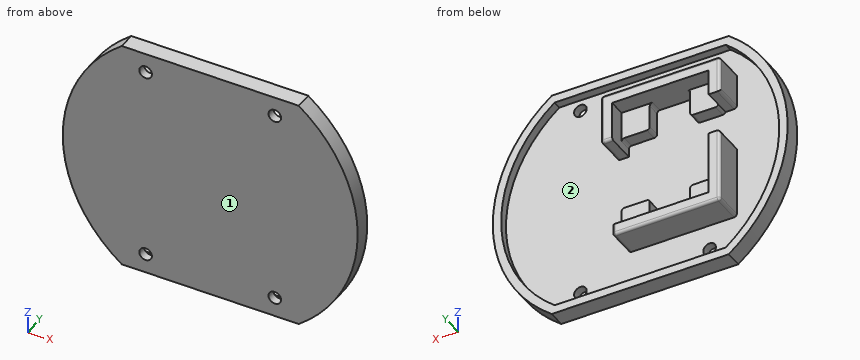
from build123d import *

# Parameters (mm, degrees)
A_BASE_T42_OUTLINE_R       = 2.2479
A_BASE_T42_OUTLINE_R_2     = 1
A_BASE_T42_DEPTH           = 3
OUTER_BRIM_DEPTH           = 3
SKETCH5_W                  = 3
SKETCH5_H                  = 15
SKETCH5_W_2                = 15
SKETCH5_H_2                = 3
BASE_SUPPORTS_DEPTH        = 3
BASE_SUPPORTS_CHAMFER_SIZE = 3
COVER_START                = -3
SKETCH6_R                  = 1
COVER_DEPTH                = 3
SKETCH9_W                  = 15
SKETCH9_H                  = 6
SKETCH9_W_2                = 6
SKETCH9_H_2                = 15
CUT_EXTRUDE1_DEPTH         = 10
SKETCH10_W                 = 10
SKETCH10_H                 = 10
BOSS_EXTRUDE1_DEPTH        = 4.6
BOSS_EXTRUDE2_DEPTH        = 10.6
FILLET1_R                  = 1


with BuildPart() as part:
    # a_base_t42: read off the stored shape, not the designer's step
    # a_base_t42 outline → a_base_t42 (new body)
    with BuildSketch(Plane(origin=(0, 0, 0), x_dir=(1, 0, 0), z_dir=(0, 1, 0))):
        with BuildLine():
            ThreePointArc((31.5, -42), (52.5, 0), (31.5, 42))
            Line((31.5, 42), (-31.5, 42))
            ThreePointArc((-31.5, 42), (-52.5, 0), (-31.5, -42))
            Line((-31.5, -42), (31.5, -42))
        make_face()
        with Locations((-23, -35)):
            Circle(A_BASE_T42_OUTLINE_R, mode=Mode.SUBTRACT)
        with Locations((23, -35)):
            Circle(A_BASE_T42_OUTLINE_R, mode=Mode.SUBTRACT)
        with Locations((-40.25, 0)):
            Circle(A_BASE_T42_OUTLINE_R_2, mode=Mode.SUBTRACT)
        with Locations((-23, 35)):
            Circle(A_BASE_T42_OUTLINE_R, mode=Mode.SUBTRACT)
        with Locations((40.25, 0)):
            Circle(A_BASE_T42_OUTLINE_R_2, mode=Mode.SUBTRACT)
        with Locations((23, 35)):
            Circle(A_BASE_T42_OUTLINE_R, mode=Mode.SUBTRACT)
    extrude(amount=A_BASE_T42_DEPTH)

    # Sketch1 → Outer Brim (add)
    with BuildSketch(Plane(origin=(0, 3, 0), x_dir=(1, 0, 0), z_dir=(0, 1, 0))):
        with BuildLine():
            Line((-31.5, -42), (31.5, -42))
            ThreePointArc((31.5, -42), (52.5, 0), (31.5, 42))
            Line((31.5, 42), (-31.5, 42))
            ThreePointArc((-31.5, 42), (-52.5, 0), (-31.5, -42))
        make_face()
        with BuildLine():
            Line((30.483602149, 39), (-30.483602149, 39))
            ThreePointArc((-30.483602149, 39), (-49.5, 0), (-30.483602149, -39))
            Line((-30.483602149, -39), (30.483602149, -39))
            ThreePointArc((30.483602149, -39), (49.5, 0), (30.483602149, 39))
        make_face(mode=Mode.SUBTRACT)
    extrude(amount=OUTER_BRIM_DEPTH)

    # Sketch5 → Base Supports (add)
    with BuildSketch(Plane(origin=(0, 3, 0), x_dir=(1, 0, 0), z_dir=(0, 1, 0))):
        with Locations((-34.325, -12.5)):
            Rectangle(SKETCH5_W, SKETCH5_H)
        with Locations((-34.325, 12.5)):
            Rectangle(SKETCH5_W, SKETCH5_H)
        with Locations((-25.325, -27)):
            Rectangle(SKETCH5_W_2, SKETCH5_H_2)
        with Locations((-25.325, 27)):
            Rectangle(SKETCH5_W_2, SKETCH5_H_2)
    extrude(amount=BASE_SUPPORTS_DEPTH)

    # Base Supports Chamfer
    base_supports_chamfer_edges = [part.edges().sort_by_distance(p)[0] for p in [
        (-25.325, 3, 28.5),
        (-25.325, 3, -28.5),
        (-35.825, 3, 12.5),
        (-35.825, 3, -12.5),
    ]]
    chamfer(base_supports_chamfer_edges, length=BASE_SUPPORTS_CHAMFER_SIZE - 0.0001)  # a hair under: the kernel refuses the full size

    # Sketch6 → Cover (add)
    with BuildSketch(Plane(origin=(0, 3, 0), x_dir=(1, 0, 0), z_dir=(0, 1, 0)).offset(COVER_START)):
        with Locations((-40.25, 0)):
            Circle(SKETCH6_R)
        with Locations((40.25, 0)):
            Circle(SKETCH6_R)
    extrude(amount=COVER_DEPTH)

    # Sketch9 → Cut-Extrude1 (cut)
    with BuildSketch(Plane(origin=(0, 3, 0), x_dir=(1, 0, 0), z_dir=(0, 1, 0))):
        with Locations((-25.325, 28.5)):
            Rectangle(SKETCH9_W, SKETCH9_H)
        with Locations((-35.825, 12.5)):
            Rectangle(SKETCH9_W_2, SKETCH9_H_2)
        with Locations((-35.825, -12.5)):
            Rectangle(SKETCH9_W_2, SKETCH9_H_2)
        with Locations((-25.325, -28.5)):
            Rectangle(SKETCH9_W, SKETCH9_H)
    extrude(amount=CUT_EXTRUDE1_DEPTH, mode=Mode.SUBTRACT)

    # Sketch10 → Boss-Extrude1 (add)
    with BuildSketch(Plane(origin=(0, 3, 0), x_dir=(1, 0, 0), z_dir=(0, 1, 0))):
        with Locations((-23.7, 16.95)):
            Rectangle(SKETCH10_W, SKETCH10_H)
        with Locations((0.7, 16.95)):
            Rectangle(SKETCH10_W, SKETCH10_H)
        with Locations((0.7, -19.95)):
            Rectangle(SKETCH10_W, SKETCH10_H)
        with Locations((-23.7, -19.95)):
            Rectangle(SKETCH10_W, SKETCH10_H)
    extrude(amount=BOSS_EXTRUDE1_DEPTH)

    # Sketch11 → Boss-Extrude2 (add)
    with BuildSketch(Plane(origin=(0, 3, 0), x_dir=(1, 0, 0), z_dir=(0, 1, 0))):
        Polygon((-28.7, 21.95), (-28.7, -0.7), (-32.7, -0.7), (-32.7, 25.95), (5.7, 25.95), (5.7, 21.95), align=None)
        Polygon((-28.7, -24.95), (-28.7, -15.7), (-32.7, -15.7), (-32.7, -28.95), (9.7, -28.95), (9.7, -10.95), (5.7, -10.95), (5.7, -24.95), align=None)
    extrude(amount=BOSS_EXTRUDE2_DEPTH)

    # Fillet1
    # the kernel refuses this fillet: 1 mm, written as the material it adds along each edge
    with BuildSketch(Plane(origin=(-18.7, 0.5, 24.95), x_dir=(1, 0, 0), z_dir=(0, 1, 0)), Plane(origin=(-4.3, 0.5, 24.95), x_dir=(0, 0, -1), z_dir=(0, 1, 0)), Plane(origin=(5.7, 0.5, 14.95), x_dir=(0, 0, -1), z_dir=(0, 1, 0)), Plane(origin=(-4.3, 0.5, -21.95), x_dir=(-1, 0, 0), z_dir=(0, 1, 0)), Plane(origin=(-18.7, 0.5, -21.95), x_dir=(0, 0, 1), z_dir=(0, 1, 0)), Plane(origin=(-28.7, 0.5, -11.95), x_dir=(0, 0, 1), z_dir=(0, 1, 0))) as fillet1_piece_1:
        with BuildLine():
            CenterArc((FILLET1_R, FILLET1_R), FILLET1_R, 180, 90)
            Line((0, FILLET1_R), (0, 0))
            Line((0, 0), (FILLET1_R, 0))
        make_face()
    extrude(amount=7.1)
    # the kernel refuses this fillet: 1 mm, written as the material it takes off along each edge
    with BuildSketch(Plane(origin=(-31.7, 12.6, 27.95), x_dir=(0, 1, 0), z_dir=(-1, 0, 0))) as fillet1_2_piece_1_section:
        Polygon((0, 0), (FILLET1_R * 1.02, 0), (FILLET1_R * 1.02, -FILLET1_R * 1.02), (0, -FILLET1_R * 1.02), align=None)
    fillet1_2_piece_1 = extrude(amount=FILLET1_R * 1.02, mode=Mode.PRIVATE)
    fillet1_2_piece_1 = fillet1_2_piece_1 - Plane(origin=(-31.7, 12.6, 27.95), x_dir=(0, -0.7071067811865475, -0.7071067811865475), z_dir=(-1, 0, 0)) * Sphere(FILLET1_R, mode=Mode.PRIVATE)
    add(fillet1_2_piece_1, mode=Mode.SUBTRACT)
    with BuildSketch(Plane(origin=(8.7, 12.6, 27.95), x_dir=(1, 0, 0), z_dir=(0, 1, 0))) as fillet1_2_piece_2_section:
        Polygon((0, 0), (FILLET1_R * 1.02, 0), (FILLET1_R * 1.02, -FILLET1_R * 1.02), (0, -FILLET1_R * 1.02), align=None)
    fillet1_2_piece_2 = extrude(amount=FILLET1_R * 1.02, mode=Mode.PRIVATE)
    fillet1_2_piece_2 = fillet1_2_piece_2 - Plane(origin=(8.7, 12.6, 27.95), x_dir=(-0.7071067811865475, 0, -0.7071067811865475), z_dir=(0, 1, 0)) * Sphere(FILLET1_R, mode=Mode.PRIVATE)
    add(fillet1_2_piece_2, mode=Mode.SUBTRACT)
    with BuildSketch(Plane(origin=(8.7, 12.6, 11.95), x_dir=(0, 1, 0), z_dir=(0, 0, -1))) as fillet1_2_piece_3_section:
        Polygon((0, 0), (FILLET1_R * 1.02, 0), (FILLET1_R * 1.02, FILLET1_R * 1.02), (0, FILLET1_R * 1.02), align=None)
    fillet1_2_piece_3 = extrude(amount=FILLET1_R * 1.02, mode=Mode.PRIVATE)
    fillet1_2_piece_3 = fillet1_2_piece_3 - Plane(origin=(8.7, 12.6, 11.95), x_dir=(-0.7071067811865475, -0.7071067811865475, 0), z_dir=(0, 0, -1)) * Sphere(FILLET1_R, mode=Mode.PRIVATE)
    add(fillet1_2_piece_3, mode=Mode.SUBTRACT)
    with BuildSketch(Plane(origin=(4.7, 12.6, -24.95), x_dir=(1, 0, 0), z_dir=(0, 0, -1))) as fillet1_2_piece_4_section:
        Polygon((0, 0), (FILLET1_R * 1.02, 0), (FILLET1_R * 1.02, -FILLET1_R * 1.02), (0, -FILLET1_R * 1.02), align=None)
    fillet1_2_piece_4 = extrude(amount=FILLET1_R * 1.02, mode=Mode.PRIVATE)
    fillet1_2_piece_4 = fillet1_2_piece_4 - Plane(origin=(4.7, 12.6, -24.95), x_dir=(-0.7071067811865475, -0.7071067811865475, 0), z_dir=(0, 0, -1)) * Sphere(FILLET1_R, mode=Mode.PRIVATE)
    add(fillet1_2_piece_4, mode=Mode.SUBTRACT)
    with BuildSketch(Plane(origin=(-31.7, 12.6, -24.95), x_dir=(0, 1, 0), z_dir=(0, 0, -1))) as fillet1_2_piece_5_section:
        Polygon((0, 0), (FILLET1_R * 1.02, 0), (FILLET1_R * 1.02, -FILLET1_R * 1.02), (0, -FILLET1_R * 1.02), align=None)
    fillet1_2_piece_5 = extrude(amount=FILLET1_R * 1.02, mode=Mode.PRIVATE)
    fillet1_2_piece_5 = fillet1_2_piece_5 - Plane(origin=(-31.7, 12.6, -24.95), x_dir=(0.7071067811865475, -0.7071067811865475, 0), z_dir=(0, 0, -1)) * Sphere(FILLET1_R, mode=Mode.PRIVATE)
    add(fillet1_2_piece_5, mode=Mode.SUBTRACT)
    with BuildSketch(Plane(origin=(-32.7, 13.6, 13.2), x_dir=(1, 0, 0), z_dir=(0, 0, 1))) as fillet1_2_piece_6:
        with BuildLine():
            CenterArc((FILLET1_R, -FILLET1_R), FILLET1_R, 90, 90)
            Line((0, -FILLET1_R), (0, 0))
            Line((0, 0), (FILLET1_R, 0))
        make_face()
    extrude(amount=14.75, mode=Mode.SUBTRACT)
    with BuildSketch(Plane(origin=(-31.7, 13.6, 28.95), x_dir=(0, 0, -1), z_dir=(1, 0, 0))) as fillet1_2_piece_7:
        with BuildLine():
            CenterArc((FILLET1_R, -FILLET1_R), FILLET1_R, 90, 90)
            Line((0, -FILLET1_R), (0, 0))
            Line((0, 0), (FILLET1_R, 0))
        make_face()
    extrude(amount=40.4, mode=Mode.SUBTRACT)
    with BuildSketch(Plane(origin=(9.7, 13.6, 27.95), x_dir=(-1, 0, 0), z_dir=(0, 0, -1))) as fillet1_2_piece_8:
        with BuildLine():
            CenterArc((FILLET1_R, -FILLET1_R), FILLET1_R, 90, 90)
            Line((0, -FILLET1_R), (0, 0))
            Line((0, 0), (FILLET1_R, 0))
        make_face()
    extrude(amount=16, mode=Mode.SUBTRACT)
    with BuildSketch(Plane(origin=(5.7, 13.6, -24.95), x_dir=(-1, 0, 0), z_dir=(0, 0, 1))) as fillet1_2_piece_9:
        with BuildLine():
            CenterArc((FILLET1_R, FILLET1_R), FILLET1_R, 180, 90)
            Line((0, FILLET1_R), (0, 0))
            Line((0, 0), (FILLET1_R, 0))
        make_face()
    extrude(amount=5.5, mode=Mode.SUBTRACT)
    with BuildSketch(Plane(origin=(-31.7, 13.6, -25.95), x_dir=(0, 0, 1), z_dir=(1, 0, 0))) as fillet1_2_piece_10:
        with BuildLine():
            CenterArc((FILLET1_R, FILLET1_R), FILLET1_R, 180, 90)
            Line((0, FILLET1_R), (0, 0))
            Line((0, 0), (FILLET1_R, 0))
        make_face()
    extrude(amount=36.4, mode=Mode.SUBTRACT)
    with BuildSketch(Plane(origin=(-32.7, 13.6, 3.2), x_dir=(1, 0, 0), z_dir=(0, 0, -1))) as fillet1_2_piece_11:
        with BuildLine():
            CenterArc((FILLET1_R, FILLET1_R), FILLET1_R, 180, 90)
            Line((0, FILLET1_R), (0, 0))
            Line((0, 0), (FILLET1_R, 0))
        make_face()
    extrude(amount=28.15, mode=Mode.SUBTRACT)
    with BuildSketch(Plane(origin=(-32.7, 3, 0.7), x_dir=(1, 0, 0), z_dir=(0, 1, 0)), Plane(origin=(-32.7, 3, 15.7), x_dir=(0, 0, 1), z_dir=(0, 1, 0))) as fillet1_2_piece_12:
        with BuildLine():
            CenterArc((FILLET1_R, FILLET1_R), FILLET1_R, 180, 90)
            Line((0, FILLET1_R), (0, 0))
            Line((0, 0), (FILLET1_R, 0))
        make_face()
    extrude(amount=13.1, mode=Mode.SUBTRACT)
    with BuildSketch(Plane(origin=(-32.7, 3, -25.95), x_dir=(0, 0, 1), z_dir=(0, 1, 0)), Plane(origin=(5.7, 3, -25.95), x_dir=(-1, 0, 0), z_dir=(0, 1, 0)), Plane(origin=(9.7, 3, 10.95), x_dir=(-1, 0, 0), z_dir=(0, 1, 0)), Plane(origin=(9.7, 3, 28.95), x_dir=(0, 0, -1), z_dir=(0, 1, 0)), Plane(origin=(-32.7, 3, 28.95), x_dir=(1, 0, 0), z_dir=(0, 1, 0))) as fillet1_2_piece_13:
        with BuildLine():
            CenterArc((FILLET1_R, FILLET1_R), FILLET1_R, 180, 90)
            Line((0, FILLET1_R), (0, 0))
            Line((0, 0), (FILLET1_R, 0))
        make_face()
    extrude(amount=9.6, mode=Mode.SUBTRACT)
    with BuildSketch(Plane(origin=(-28.7, 3, 14.95), x_dir=(0, 0, 1), z_dir=(0, 1, 0))) as fillet1_2_piece_14:
        with BuildLine():
            CenterArc((1, 0.968245837), FILLET1_R, 180, 75.522487814)
            Line((0, 0.968245837), (0, 0))
            Line((0, 0), (0.75, 0))
        make_face()
    extrude(amount=7.020614591, mode=Mode.SUBTRACT)
    with BuildSketch(Plane(origin=(-18.7, 3, 14.95), x_dir=(-1, 0, 0), z_dir=(0, 1, 0)), Plane(origin=(-4.3, 3, 14.95), x_dir=(0, 0, 1), z_dir=(0, 1, 0)), Plane(origin=(5.7, 3, -11.95), x_dir=(0, 0, -1), z_dir=(0, 1, 0)), Plane(origin=(-4.3, 3, -11.95), x_dir=(1, 0, 0), z_dir=(0, 1, 0))) as fillet1_2_piece_15:
        with BuildLine():
            CenterArc((FILLET1_R, FILLET1_R), FILLET1_R, 180, 90)
            Line((0, FILLET1_R), (0, 0))
            Line((0, 0), (FILLET1_R, 0))
        make_face()
    extrude(amount=7.1, mode=Mode.SUBTRACT)
    with BuildSketch(Plane(origin=(-18.7, 3, -11.95), x_dir=(-1, 0, 0), z_dir=(0, 1, 0))) as fillet1_2_piece_16:
        with BuildLine():
            CenterArc((FILLET1_R, -FILLET1_R), FILLET1_R, 90, 90)
            Line((0, -FILLET1_R), (0, 0))
            Line((0, 0), (FILLET1_R, 0))
        make_face()
    extrude(amount=7.1, mode=Mode.SUBTRACT)
    with BuildSketch(Plane(origin=(8.7, 13.6, 10.95), x_dir=(0, 0, 1), z_dir=(-1, 0, 0))) as fillet1_2_piece_17:
        with BuildLine():
            CenterArc((FILLET1_R, -FILLET1_R), FILLET1_R, 90, 90)
            Line((0, -FILLET1_R), (0, 0))
            Line((0, 0), (FILLET1_R, 0))
        make_face()
    extrude(amount=5.5, mode=Mode.SUBTRACT)


solid = part.part
Geometry check sheet. Reference: the model listing, model coordinates, mm. Face numbers are marked on the shaded views. Round coordinates to 2 decimals unless told otherwise and drop trailing zeros. Write each loop counter-clockwise with the first axis right and the second up, starting at its lowest first coordinate (ties: lowest second). Pieces come first, ordered by that corner, then holes. Notation, with made-up numbers: (77.25, 10) - (123.25, 10) arc R27 ccw to (123.25, 40) - close; hole circle Ø8 at (49.25, -3). An arc over 180 degrees is marked (long way). One line per item, written item: value.
1. Cross-section at B-B on x = 23. Record the boundary of the cut face in (y, z), and give its area (3 significant figures).
The answers:
outline: (0, -42) - (6, -42) - (6, -39) - (3, -39) - (3, -37.25) - (0, -37.25) - close; (0, -32.75) - (3, -32.75) - (3, 32.75) - (0, 32.75) - close; (0, 37.25) - (3, 37.25) - (3, 39) - (6, 39) - (6, 42) - (0, 42) - close
area: 243 mm^2
2. Scan lines: L1, parallel to Z at x = 23, y = 2; L2, parallel to Z at x = 4, y = 5.5; L3, parallel to Z at x = -8.5, y = 11. Record each from-to range of solid material in increasing order.
The answers:
L1: z = -42 to -37.25, -32.75 to 32.75, 37.25 to 42
L2: z = -42 to -39, -25.95 to -11.95, 14.95 to 28.95, 39 to 42
L3: z = -25.95 to -21.95, 24.95 to 28.95
3. Depth check by flat-ended pin: pin 1 Ø5 at (y, z) = (7.5, -14) entering from -X; pin 2 Ø4 at (y, z) = (6, -12.5) entering from +X; pin 3 Ø1 at (y, z) = (2, -26.5) entering from +X. Enter the tip coordinate at first touch or a pass-through.
The answers:
pin 1: stops at x = -51.11
pin 2: stops at x = 51.44
pin 3: stops at x = 45.61
4. Cross-section at C-C on y = 4.75. Give the number of separate pieces and of enclosed holes in the cut face, and give its area (3 significant figures).
The answers:
separate pieces: 3
enclosed holes: 1
area: 1,840 mm^2
5. Cross-section at D-D on z = 35. Record the boundary of the cut face in (x, y).
The answers:
outline: (-39.13, 0) - (-25.25, 0) - (-25.25, 3) - (-35, 3) - (-35, 6) - (-39.13, 6) - close; (-20.75, 0) - (20.75, 0) - (20.75, 3) - (-20.75, 3) - close; (25.25, 0) - (39.13, 0) - (39.13, 6) - (35, 6) - (35, 3) - (25.25, 3) - close
6. Cross-section at A-A on y = 9.75. Record the boundary of the cut face in (x, z).
The answers:
outline: (-32.7, -24.95) arc R1 ccw to (-31.7, -25.95) - (4.7, -25.95) arc R1 ccw to (5.7, -24.95) - (5.7, -21.95) - (-28.7, -21.95) - (-28.7, 0.7) - (-31.7, 0.7) arc R1 ccw to (-32.7, -0.3) - close; (-32.7, 16.7) arc R1 ccw to (-31.7, 15.7) - (-28.7, 15.7) - (-28.7, 24.95) - (5.7, 24.95) - (5.7, 10.95) - (8.7, 10.95) arc R1 ccw to (9.7, 11.95) - (9.7, 27.95) arc R1 ccw to (8.7, 28.95) - (-31.7, 28.95) arc R1 ccw to (-32.7, 27.95) - close
7. Mould release check, pull along Z, two halves, no side actions. Record for the marked faces 1 and 2: released by +Z, released by -Z, zero draft, split by the parting line, or undercut.
The answers:
face 1: zero draft
face 2: undercut
